Work out the finished part from the listing and answer in its coordinate system (mm). A direction names the side the tool comes from. Coordinates: 2 decimals unless noted, no trailing zeros. Order: outer loops, then holes, each group sorted by start corner. A loop starts at its lowest first (then second) coordinate and runs counter-clockwise, first axis right, second up. Notation, with made-up numbers: M 89,80 L 125,80 A7 ccw 125,93 Z; hole C 43.5,-25 d9. An arc over 180 degrees is marked long. Use a Markdown table: item, result.
from build123d import *

# Parameters (mm, degrees)
C_CHANNEL_80_X_8_1_DEPTH = 800
SKETCH12_W               = 32
SKETCH12_H               = 59
BOSS_EXTRUDE1_DEPTH      = 8


with BuildPart() as part:
    # Sketch11 → C channel 80 X 8(1) (new body)
    with BuildSketch(Plane.YZ.offset(-400)):
        Polygon((0, -37.5), (0, 37.5), (40, 37.5), (40, 29.5), (8, 29.5), (8, -29.5), (40, -29.5), (40, -37.5), align=None)
    extrude(amount=C_CHANNEL_80_X_8_1_DEPTH)

    # Sketch12 → Boss-Extrude1 (add)
    with BuildSketch(Plane.XZ):
        with Locations((-416, 0)):
            Rectangle(SKETCH12_W, SKETCH12_H)
        with Locations((416, 0)):
            Rectangle(SKETCH12_W, SKETCH12_H)
    extrude(amount=-BOSS_EXTRUDE1_DEPTH)


solid = part.part
1. Flat-ended cylindrical pins translate along their axes: P1, Ø4, axis at x = -412.5, y = 3.5, coming from the -Z side; P2, Ø6.5, axis at y = 20, z = 34.5, coming from the +X side; P3, Ø9, axis at y = 18, z = -34, coming from the -X side; P4, Ø2, axis at x = -301, z = 21, coming from the -Y side. Find the tip coordinate at first contact, or state that the pin passes through.
Answers below:
| item | result |
|---|---|
| P1 | z = -29.5 |
| P2 | x = 400 |
| P3 | x = -400 |
| P4 | y = 0 |
2. For faces 5 (the face through (-6, 20, 37.5)), 6 (the face through (-6, 24, 29.5)), determine the directions among +Z, -Z, +X, -X, +Y, -Y from which every point of the face is accessible in a straight line to the end or side of a thin tool.
Answers below:
| item | result |
|---|---|
| face 5 | +Z, +X, -X, +Y, -Y |
| face 6 | +X, -X, +Y |
3. Section A-A on y = 28 is taken. Determine the outline of the cut face in (x, z).
Answers below:
| item | result |
|---|---|
| outline | M -400,-37.5 L 400,-37.5 L 400,-29.5 L -400,-29.5 Z; M -400,29.5 L 400,29.5 L 400,37.5 L -400,37.5 Z |
4. Section C-C on z = -13 is taken. Determine the outline of the cut face in (x, y).
Answers below:
| item | result |
|---|---|
| outline | M -432,0 L 432,0 L 432,8 L -432,8 Z |
5. For a pull along Z with two mould halves and no side action, classify faces 1 (the face through (-6, 8, 0)), 2 (the face through (-6, 24, -29.5)), 3 (the face through (-6, 20, -37.5)), 4 (the face through (-6, 0, 1)) as +Z half, -Z half, draft (parallel to the pull), parting line (faces both ways), or undercut.
Answers below:
| item | result |
|---|---|
| face 1 | undercut |
| face 2 | undercut |
| face 3 | -Z half |
| face 4 | draft |
6. Find the intervals of material crossed by probe 1 along Z at (x, y) = (389, 29.5); probe 2 along Y at (x, z) = (204, -17), in increasing order.
Answers below:
| item | result |
|---|---|
| probe 1 | -37.5 to -29.5, 29.5 to 37.5 |
| probe 2 | 0 to 8 |
7. Section B-B on x = 329 is taken. Determine the outline of the cut face in (y, z), then the cut area to 3 significant figures.
Answers below:
| item | result |
|---|---|
| outline | M 0,-37.5 L 40,-37.5 L 40,-29.5 L 8,-29.5 L 8,29.5 L 40,29.5 L 40,37.5 L 0,37.5 Z |
| area | 1,110 mm² |
